CAD build for the part. Positions are in the model's coordinates, mm. A direction names the side the tool comes from. Round coordinates to 2 decimals unless told otherwise and drop trailing zeros. Order: outer loops, then holes, each group sorted by start corner. A loop starts at its lowest first (then second) coordinate and runs counter-clockwise, first axis right, second up.
```python
from build123d import *

# Parameters (mm, degrees)
MAINPLATEEXTRUDE_DEPTH = 374.65
FLANGECUT_DEPTH        = 107.95
SKETCH3_W              = 74.5998
SKETCH3_H              = 349.25
CUT_EXTRUDE2_DEPTH     = 1.5875


with BuildPart() as part:
    # Sketch1 → MainPlateExtrude (new body)
    with BuildSketch(Plane(origin=(0, 0, 0), x_dir=(1, 0, 0), z_dir=(0, 1, 0))):
        with BuildLine():
            Line((-47.61865, -52.38115), (-41.26865, -52.38115))
            Line((-41.26865, -52.38115), (-41.26865, -53.96865))
            Line((-41.26865, -53.96865), (-47.61865, -53.96865))
            ThreePointArc((-47.61865, -53.96865), (-50.424980038, -52.806230038), (-51.5874, -49.9999))
            Line((-51.5874, -49.9999), (-51.5874, 49.9999))
            ThreePointArc((-51.5874, 49.9999), (-50.424980038, 52.806230038), (-47.61865, 53.96865))
            Line((-47.61865, 53.96865), (-41.26865, 53.96865))
            Line((-41.26865, 53.96865), (-41.26865, 52.38115))
            Line((-41.26865, 52.38115), (-47.61865, 52.38115))
            ThreePointArc((-47.61865, 52.38115), (-49.302448023, 51.683698023), (-49.9999, 49.9999))
            Line((-49.9999, 49.9999), (-49.9999, -49.9999))
            ThreePointArc((-49.9999, -49.9999), (-49.302448023, -51.683698023), (-47.61865, -52.38115))
        make_face()
    extrude(amount=MAINPLATEEXTRUDE_DEPTH)

    # Sketch2 → FlangeCut (cut)
    with BuildSketch(Plane.XY.offset(53.96865)):
        Polygon((-41.26865, 95.25), (-47.61865, 88.9), (-47.61865, 63.5), (-41.26865, 57.15), align=None)
        Polygon((-41.26865, 6.35), (-47.61865, 0), (-41.26865, 0), align=None)
        Polygon((-41.26865, 228.6), (-47.61865, 222.25), (-47.61865, 152.4), (-41.26865, 146.05), align=None)
        Polygon((-41.26865, 317.5), (-47.61865, 311.15), (-47.61865, 285.75), (-41.26865, 279.4), align=None)
        Polygon((-41.26865, 374.65), (-47.61865, 374.65), (-41.26865, 368.3), align=None)
    extrude(amount=-FLANGECUT_DEPTH, mode=Mode.SUBTRACT)

    # Sketch3 → Cut-Extrude2 (cut)
    with BuildSketch(Plane.ZY.offset(51.5874)):
        with Locations((0, 187.325)):
            Rectangle(SKETCH3_W, SKETCH3_H)
    extrude(amount=-CUT_EXTRUDE2_DEPTH, mode=Mode.SUBTRACT)


solid = part.part
```
1. Mould opens along Z. For faces 1 (the face through (-44, 31, 52.381)), 2 (the face through (-44, 254, -53.969)), 3 (the face through (-44, 342, 53.969)), 4 (the face through (-44.4, 3.22, -53.16)) say: released by +Z, released by -Z, zero draft, split by the parting line, or undercut.
2. Cut at C-C, the plane x = -45. Give the number of separate pieces and of enclosed holes in the cut face, and give its area (3 significant figures).
3. Pin check, flat tips, straight feed: P1, Ø1.7, axis at y = 302, z = -53.5, coming from the +X side; P2, Ø1.7, axis at x = -50.5, y = 141, coming from the -Z side; P3, Ø6, axis at y = 196, z = 37.5, coming from the +X side. Stop position of each tip, or through.
4. Drill centre lines: line 1 (Z direction, x = -44, y = 279); line 2 (Z direction, x = -50.75, y = 129.5); line 3 (Y direction, x = -50.25, z = -23.5). Where is each one in solid material? Low to high.
5. Cut at A-A, the plane z = -15.5. Write the cut outline in (x, y).
6. Tool access for faces 5 (the face through (-44, 120, 52.381)), 6 (the face through (-44.4, 314.37, 53.19)), 7 (the face through (-44.4, 3.22, 53.19)): list every direction of +Z, -Z, +X, -X, +Y, -Y with a clear straight run to the whole face (end or side of a thin tool).
7. Cut at B-B, the plane y = 202.5. Write the cut outline in (x, z).
8. Cut at D-D, the plane y = 46.5. Write the cut outline in (x, z), and give its area (3 significant figures).
Outcome:
1. face 1: undercut
1. face 2: released by -Z
1. face 3: released by +Z
1. face 4: zero draft
2. separate pieces: 8
2. enclosed holes: 0
2. area: 740 mm2
3. P1: stops at x = -47.62
3. P2: stops at z = -53.41
3. P3: stops at x = -50
4. line 1: z = -53.97 to -52.38, 52.38 to 53.97
4. line 2: z = -52.44 to -37.3, 37.3 to 52.44
4. line 3: y = 0 to 12.7, 361.95 to 374.65
5. outline: (-51.59, 0) - (-50, 0) - (-50, 12.7) - (-51.59, 12.7) - close; (-51.59, 361.95) - (-50, 361.95) - (-50, 374.65) - (-51.59, 374.65) - close
6. face 5: +X, +Y, -Y
6. face 6: +Z, -Z, +X
6. face 7: +Z, -Z, +X, -Y
7. outline: (-51.59, -50) arc R3.97 ccw to (-47.62, -53.97) - (-47.62, -52.38) arc R2.38 cw to (-50, -50) - (-50, -37.3) - (-51.59, -37.3) - close; (-51.59, 37.3) - (-50, 37.3) - (-50, 50) arc R2.38 cw to (-47.62, 52.38) - (-47.62, 53.97) arc R3.97 ccw to (-51.59, 50) - close
8. outline: (-51.59, -50) arc R3.97 ccw to (-47.62, -53.97) - (-41.27, -53.97) - (-41.27, -52.38) - (-47.62, -52.38) arc R2.38 cw to (-50, -50) - (-50, -37.3) - (-51.59, -37.3) - close; (-51.59, 37.3) - (-50, 37.3) - (-50, 50) arc R2.38 cw to (-47.62, 52.38) - (-41.27, 52.38) - (-41.27, 53.97) - (-47.62, 53.97) arc R3.97 ccw to (-51.59, 50) - close
8. area: 76.3 mm2
